Autodesk Inventor part; units mm, degrees
ref_plane "YZ Plane" through (0, 0, 0) normal (1, 0, 0) x (0, 1, 0)
ref_plane "XZ Plane" through (0, 0, 0) normal (0, 1, 0) x (-1, 0, 0)
ref_plane "XY Plane" through (0, 0, 0) normal (0, 0, 1) x (1, 0, 0)
sketch "スケッチ1" plane through (0, 0, 0) normal (0, 0, 1) x (1, 0, 0)
  circle A0 centre (0, 0) radius 13.85
  dimension "d0" = 27.7
extrude "押し出し1" add sketch "スケッチ1" along normal blind 37.8
sketch "スケッチ2" plane through (0, 0, 37.8) normal (0, 0, 1) x (1, 0, 0)
  circle A0 centre (0, 0) radius 5
  dimension "d3" = 10
extrude "押し出し2" add sketch "スケッチ2" along normal blind 2.6
sketch "スケッチ3" plane through (0, 0, 40.4) normal (0, 0, 1) x (1, 0, 0)
  circle A0 centre (0, 0) radius 1.15
  dimension "d6" = 2.3
extrude "押し出し3" add sketch "スケッチ3" along normal blind 13.8
sketch "スケッチ4" plane through (0, 0, 0) normal (0, 0, -1) x (-1, 0, 0)
  circle A0 centre (0, 0) radius 1.15
  circle A1 centre (0, 0) radius 5
  dimension "d9" = 10
extrude "押し出し4" add sketch "スケッチ4" along normal blind 2.6
extrude "押し出し5" add sketch "スケッチ4" along normal blind 2.8 contours A0
sketch "スケッチ5" plane through (0, 0, 37.8) normal (0, 0, 1) x (1, 0, 0)
  circle A0 centre (-8, 0) radius 1.3
  circle A1 centre (8, 0) radius 1.3
  line L0 (-8, 0) -> (8, 0)
  point P0 (0, 0)
  point P1 (0, 0)
  dimension "d14" = 2.6
  dimension "d15" = 2.6
  dimension "d16" = 16
  dimension "d17" = 8
hole "穴1" at (-8, 0, 37.8) at (8, 0, 37.8) direction (0, 0, -1) diameter 3 depth 8 tip angle 118
properties part number "マブチモーター　RS-380PH"
Verification items for the finished model (mm, model axes). A direction names the side the tool comes from. Coordinates: 2 decimals unless noted, no trailing zeros. Order: outer loops, then holes, each group sorted by start corner. A loop starts at its lowest first (then second) coordinate and runs counter-clockwise, first axis right, second up. Notation, with made-up numbers: (16.5, 26) -> (53.5, 26) arc R13 ccw to (53.5, 48) -> close; hole circle Ø9 at (25.5, 64). An arc over 180 degrees is marked (long way). Put each result on its own line as item: value. Start each with the question number.
1. Cross-section at B-B, the plane x = 0. Record the boundary of the cut face in (y, z), then the cut area to 3 significant figures.
2. Cross-section at A-A, the plane z = 37. Record the boundary of the cut face in (x, y), then the cut area to 3 significant figures.
3. Access from +Z, -Z, +X, -X, +Y, -Y to the whole of each face (thin tool, end or side, straight path). Record for faces 4 (the cylindrical face through (1.08, 4.88, -1.28)), 5 (the flat face through (0, 0, -2.8)), 6 (the flat face through (6, 0, 37.8)).
4. Material ranges on L1, parallel to Z at x = -5.75, y = -12.5; L2, parallel to Z at x = -1, y = 4.75; L3, parallel to Y at x = -8, z = 34, recorded low to high. Write a range as [from, to].
5. Cross-section at D-D, the plane y = 5.75. Record the boundary of the cut face in (x, z), then the cut area to 3 significant figures.
6. Mould release check, pull along Y, two halves, no side actions. Record for faces 1 (the cylindrical face through (13.21, -4.16, 18.64)), 2 (the conical face through (-8.231, -0.12, 29.055)), 3 (the flat face through (0, 0, 54.2)): released by +Y, released by -Y, zero draft, split by the parting line, or undercut.
7. Cross-section at C-C, the plane z = 45. Record the boundary of the cut face in (x, y), then the cut area to 3 significant figures.
8. Go/stop test with flat-tipped pins: pin 1 Ø6 at (x, y) = (9, -9.5) entering from +Z; pin 2 Ø2.5 at (x, y) = (-8, 0) entering from +Z; pin 3 Ø2.5 at (x, y) = (8, 0) entering from -Z. Record where each tip stops, or that it passes through.
Computed:
1. outline: (-13.85, 0) -> (-5, 0) -> (-5, -2.6) -> (-1.15, -2.6) -> (-1.15, -2.8) -> (1.15, -2.8) -> (1.15, -2.6) -> (5, -2.6) -> (5, 0) -> (13.85, 0) -> (13.85, 37.8) -> (5, 37.8) -> (5, 40.4) -> (1.15, 40.4) -> (1.15, 54.2) -> (-1.15, 54.2) -> (-1.15, 40.4) -> (-5, 40.4) -> (-5, 37.8) -> (-13.85, 37.8) -> close
1. area: 1,130 mm2
2. outline: circle Ø27.7 at (0, 0); hole circle Ø3 at (-8, 0); hole circle Ø3 at (8, 0)
2. area: 588 mm2
3. face 4: -Z
3. face 5: -Z, +X, -X, +Y, -Y
3. face 6: +Z
4. L1: [0, 37.8]
4. L2: [-2.6, 40.4]
4. L3: [-11.31, -1.5], [1.5, 11.31]
5. outline: (-12.6, 0) -> (12.6, 0) -> (12.6, 37.8) -> (-12.6, 37.8) -> close
5. area: 953 mm2
6. face 1: split by the parting line
6. face 2: undercut
6. face 3: zero draft
7. outline: circle Ø2.3 at (0, 0)
7. area: 4.15 mm2
8. pin 1: z = 37.8
8. pin 2: z = 29.65
8. pin 3: z = 0
